Job drawing, mm, ordinate dimensions from the low corner. One solid piece. Round coordinates to 2 decimals unless told otherwise and drop trailing zeros. Loops run counter-clockwise (first coordinate to the right, second up) from the corner with the lowest first, then second, coordinate; pieces in that order, holes last.
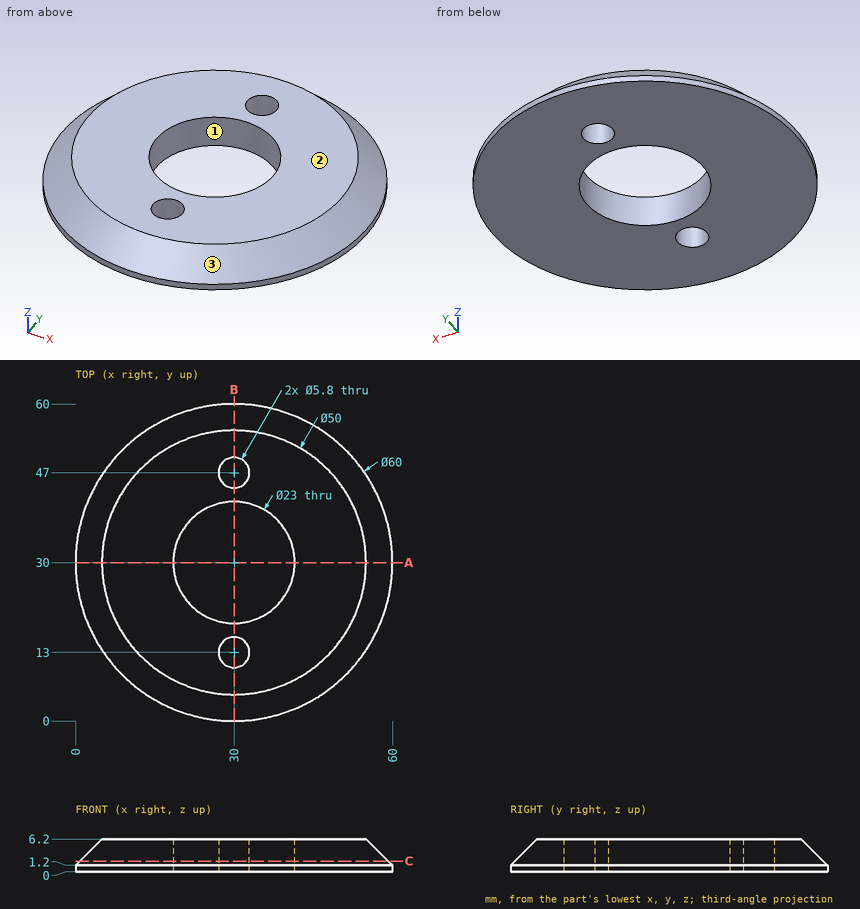
(1) Pin check, flat tip, straight feed: P1, Ø3, axis at x = 27.5, z = 5.5, coming from the +Y side. Stop position of the tip, or through.
Responses:
P1: stops at y = 57.09
(2) Slice it at C-C on z = 2. List the corners of the cut face in (x, y), plus the area to 3 significant figures.
Responses:
outline: circle Ø58.4 at (30, 30); hole circle Ø23 at (30, 30); hole circle Ø5.8 at (30, 13); hole circle Ø5.8 at (30, 47)
area: 2,210 mm2
(3) Probe line 1 (Y direction, x = 30, z = 3.75); line 2 (Y direction, x = 30, z = 4.5); line 3 (Y direction, x = 27, z = 4.25). List the from-to ranges inside material, lowest first.
Responses:
line 1: y = 2.55 to 10.1, 15.9 to 18.5, 41.5 to 44.1, 49.9 to 57.45
line 2: y = 3.3 to 10.1, 15.9 to 18.5, 41.5 to 44.1, 49.9 to 56.7
line 3: y = 3.22 to 18.9, 41.1 to 56.78
(4) Pull direction X, two halves, no side cores. Call the marked faces 1, 2 and 3: +X half, -X half, draft (parallel to the pull), parting line (faces both ways), or undercut.
Responses:
face 1: undercut
face 2: draft
face 3: parting line
(5) Slice it at B-B on x = 30. List the corners of the cut face in (y, z), plus the area to 3 significant figures.
Responses:
outline: (0, 0) - (10.1, 0) - (10.1, 6.2) - (5, 6.2) - (0, 1.2) - close; (15.9, 0) - (18.5, 0) - (18.5, 6.2) - (15.9, 6.2) - close; (41.5, 0) - (44.1, 0) - (44.1, 6.2) - (41.5, 6.2) - close; (49.9, 0) - (60, 0) - (60, 1.2) - (55, 6.2) - (49.9, 6.2) - close
area: 132 mm2
(6) Slice it at A-A on y = 30. List the corners of the cut face in (x, z).
Responses:
outline: (0, 0) - (18.5, 0) - (18.5, 6.2) - (5, 6.2) - (0, 1.2) - close; (41.5, 0) - (60, 0) - (60, 1.2) - (55, 6.2) - (41.5, 6.2) - close
